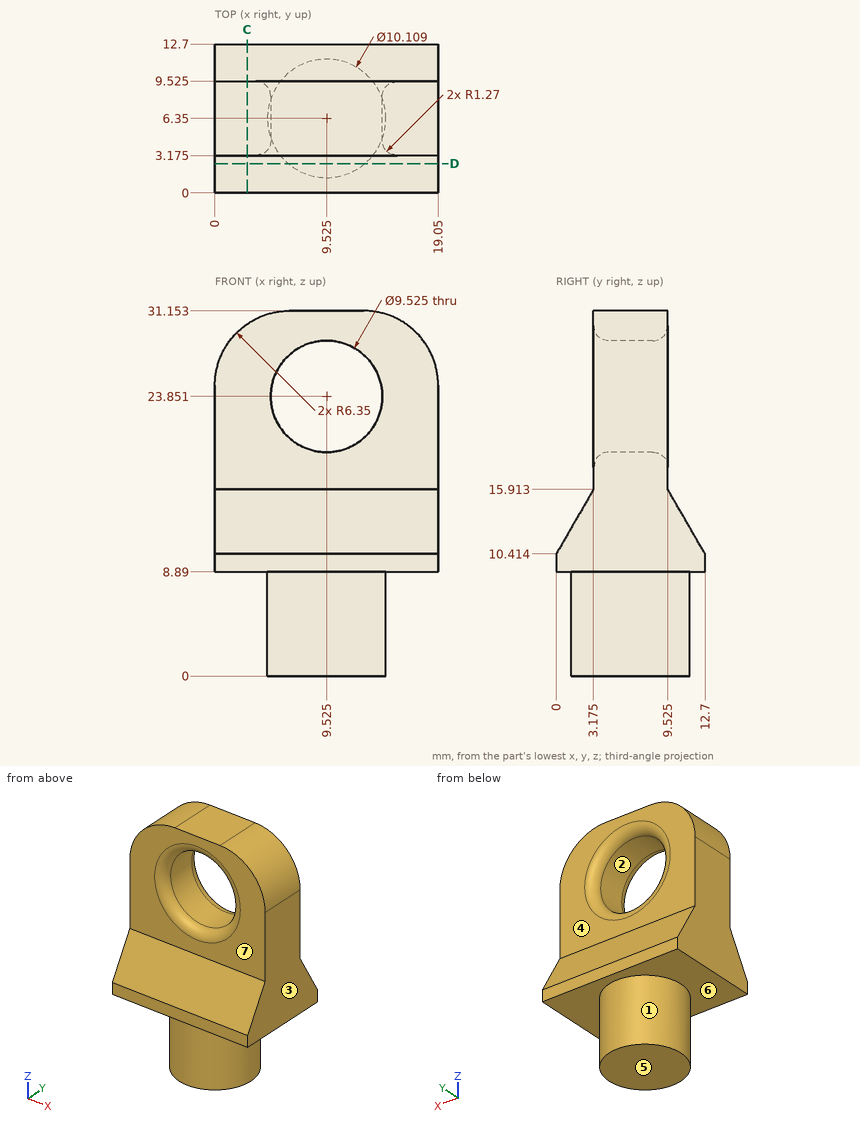
Study the drawing (mm; zero at the part's minimum x, y, z) and answer. A direction names the side the tool comes from. Give positions to 0.01 mm unless a question says otherwise; leave off trailing zeros. Loops run counter-clockwise (first coordinate to the right, second up) from the corner with the lowest first, then second, coordinate; pieces in that order, holes last. Notation, with made-up numbers: (-9, 39) - (16, 39) arc R19 cw to (16, 73) - close; hole circle Ø10 at (-16, 6.25). An arc over 180 degrees is marked (long way). Return JSON: item names as keys, results as strings. Group by question number.
1. Straight lines are drawn through the part: line 1 (Y direction, x = 9.25, z = 4.5); line 2 (Y direction, x = 16, z = 21.5) (1 decimal); line 3 (X direction, y = 3.75, z = 24). For each, find the intervals that lie inside material, in ascending order. Write a range as [from, to].
2. Find section D-D (y = 2.5). Write down the section's boundary in (x, z).
3. Find section C-C (x = 2.75). Write down the section's boundary in (y, z) (1 decimal), then the cut area to 3 significant figures.
4. Given pin 1 Ø1.5 at (x, y) = (14.5, 9.5) entering from +Z; pin 2 Ø7.5 at (x, z) = (10.5, 27) entering from +Y (3 decimals); pin 3 Ø4 at (x, y) = (14, 5) entering from -Z; pin 4 Ø7.5 at (x, z) = (13.5, 21) entering from -Y (3 decimals), each flat-ended and moving along its own axis, determine where each tip first touches the part or whether it passes through.
5. Determine the mould class of the marked faces 1, 2, 3 and 4 for opening direction X: pulls with the +X half, pulls with the -X half, needs draft (parallel to the pull), parting line crosses it, or undercut.
6. Which of the six approach directions +Z, -Z, +X, -X, +Y, -Y give full straight-line access (tool end or side, diameter ignored) to the marked faces 5, 6 and 7?
Verdict:
{
 "1": {"line 1": "y = [1.3, 11.4]", "line 2": "y = [3.2, 9.5]", "line 3": "x = [0, 4.56], [14.49, 19.05]"},
 "2": {"outline": "(0, 8.89) - (6.25, 8.89) - (6.25, 0) - (12.8, 0) - (12.8, 8.89) - (19.05, 8.89) - (19.05, 14.74) - (0, 14.74) - close"},
 "3": {"outline": "(0, 8.9) - (12.7, 8.9) - (12.7, 10.4) - (9.5, 15.9) - (9.5, 30) - (3.2, 30) - (3.2, 15.9) - (0, 10.4) - close", "area": "161 mm^2"},
 "4": {"pin 1": "stops at z = 31.07", "pin 2": "stops at y = 9.525", "pin 3": "stops at z = 0", "pin 4": "stops at y = 3.175"},
 "5": {"face 1": "parting line crosses it", "face 2": "undercut", "face 3": "pulls with the +X half", "face 4": "needs draft"},
 "6": {"face 5": "-Z, +X, -X, +Y, -Y", "face 6": "-Z", "face 7": "+Z, +X, -X, -Y"}
}
